Here's how the part is built. I have some questions about the finished solid (model axes, mm). A direction names the side the tool comes from. Give positions to 0.01 mm unless a question says otherwise; leave off trailing zeros. Loops run counter-clockwise (first coordinate to the right, second up) from the corner with the lowest first, then second, coordinate; pieces in that order, holes last. Notation, with made-up numbers: (5, 55) - (15, 55) arc R12 cw to (15, 78) - close; hole circle Ø1 at (-30, -38.75). An arc over 180 degrees is marked (long way). Put each result on its own line as item: value. Start each with the question number.
Autodesk Inventor part; units mm, degrees
ref_plane "YZ Plane" through (0, 0, 0) normal (1, 0, 0) x (0, 1, 0)
ref_plane "XZ Plane" through (0, 0, 0) normal (0, 1, 0) x (-1, 0, 0)
ref_plane "XY Plane" through (0, 0, 0) normal (0, 0, 1) x (1, 0, 0)
sketch "スケッチ1" plane through (0, 0, 0) normal (0, 0, 1) x (1, 0, 0)
  line L0 (-7.5, -5) -> (7.5, -5)
  line L1 (7.5, -5) -> (7.5, 5)
  line L2 (7.5, 5) -> (-7.5, 5)
  line L3 (-7.5, 5) -> (-7.5, -5)
  line L4 (-7.5, -5) -> (7.5, 5) construction
  line L5 (7.5, -5) -> (-7.5, 5) construction
  point P0 (0, 0)
  dimension "d0" = 15
  dimension "d1" = 10
extrude "押し出し1" add sketch "スケッチ1" along normal mid plane 10
sketch "スケッチ2" plane through (-7.5, 5, 5) normal (0, 1, 0) x (1, 0, 0)
  line L0 (13, 2) -> (2, 2)
  line L1 (2, 2) -> (2, 8)
  line L2 (2, 8) -> (13, 8)
  line L3 (13, 8) -> (13, 2)
  line L4 (13, 2) -> (2, 8) construction
  line L5 (2, 2) -> (13, 8) construction
  point P0 (7.5, 5)
  dimension "d4" = 6
  dimension "d5" = 11
extrude "押し出し2" cut sketch "スケッチ2" against normal blind 10
sketch "スケッチ3" plane through (0, 0, -5) normal (0, 0, -1) x (-1, 0, 0)
  line L0 (-7.5, -5) -> (7.5, -5)
  line L1 (-7.5, 5) -> (-7.5, -5)
  line L2 (7.5, -5) -> (7.5, 5)
  point P0 (0, 0)
  point P1 (-3.5, -1.5)
  point P2 (3.5, -1.5)
  dimension "d8" = 3.5
  dimension "d9" = 4
  dimension "d10" = 4
  dimension "d11" = 3.5
hole "穴1" at (3.5, -1.5, -5) at (-3.5, -1.5, -5) direction (0, 0, 1) diameter 2.2 depth 4 tip angle 118
properties part number "sponge"
1) Suppose I cut it at B-B on z = 2.25. Please give me the cut outline in (x, y).
2) I need wall thicknesses on line 1 (X direction, y = -1.5, z = -3.7); line 2 (Z direction, x = -5, y = -3.5); line 3 (Y direction, x = -3.5, z = -4.15). Which ranges of each line are inside material? Lowest first, please.
3) Suppose I cut it at C-C on y = -1.5. Please give me the cut outline in (x, z), plus the area to 3 significant figures.
4) Suppose I cut it at A-A on x = -0.25. Please give me the cut outline in (y, z), plus the area to 3 significant figures.
5) Which directions (+Z, -Z, +X, -X, +Y, -Y) give clear straight access to the entire face, cutting with the end or side of a thin tool? Please do faces 4 (the flat face through (0, 0, -5)), 5 (the cylindrical face through (-4.59, -1.64, -3.99)), 6 (the flat face through (-5.5, 0, 0)).
6) Suppose I cut it at D-D on x = -3.5. Please give me the cut outline in (y, z), plus the area to 3 significant figures.
7) Thinking about a two-plate mould opening in Z: for faces 1 (the flat face through (0, 0, -3)), 2 (the flat face through (0, 0, 5)), 3 (the flat face through (7.5, 0, 0)), which applies, pulls with the +Z half, pulls with the -Z half, needs draft (parallel to the pull), parting line crosses it, or undercut?
8) I'm going to push a flat-ended pin straight in: P1, Ø1.8, axis at x = -3.5, y = -1.5, coming from the -Z side. Where does the tip first touch, or does it pass through?
Ans:
1. outline: (-7.5, -5) - (-5.5, -5) - (-5.5, 5) - (-7.5, 5) - close; (5.5, -5) - (7.5, -5) - (7.5, 5) - (5.5, 5) - close
2. line 1: x = -7.5 to -4.6, -2.4 to 2.4, 4.6 to 7.5
2. line 2: z = -5 to -3, 3 to 5
2. line 3: y = -5 to -2.6, -0.4 to 5
3. outline: (-7.5, -5) - (-4.6, -5) - (-4.6, -3) - (-5.5, -3) - (-5.5, 3) - (5.5, 3) - (5.5, -3) - (4.6, -3) - (4.6, -5) - (7.5, -5) - (7.5, 5) - (-7.5, 5) - close; (-2.4, -5) - (2.4, -5) - (2.4, -3) - (-2.4, -3) - close
3. area: 75.2 mm²
4. outline: (-5, -5) - (5, -5) - (5, -3) - (-5, -3) - close; (-5, 3) - (5, 3) - (5, 5) - (-5, 5) - close
4. area: 40.0 mm²
5. face 4: -Z, +X, -X, +Y, -Y
5. face 5: -Z
5. face 6: +Y, -Y
6. outline: (-5, -5) - (-2.6, -5) - (-2.6, -3) - (-5, -3) - close; (-5, 3) - (5, 3) - (5, 5) - (-5, 5) - close; (-0.4, -5) - (5, -5) - (5, -3) - (-0.4, -3) - close
6. area: 35.6 mm²
7. face 1: undercut
7. face 2: pulls with the +Z half
7. face 3: needs draft
8. P1: stops at z = 3
